Autodesk Inventor part; units mm, degrees
ref_plane "YZ Plane" through (0, 0, 0) normal (1, 0, 0) x (0, 1, 0)
ref_plane "XZ Plane" through (0, 0, 0) normal (0, 1, 0) x (-1, 0, 0)
ref_plane "XY Plane" through (0, 0, 0) normal (0, 0, 1) x (1, 0, 0)
sketch "Sketch1" plane through (0, 0, 0) normal (0, 0, 1) x (1, 0, 0)
  circle A0 centre (0, 0) radius 15.25
  circle A1 centre (0, 0) radius 17.5
  line L0 (-17.4453, -1.3829) -> (-17.4453, 0)
  line L1 (-17.9063, 7.789) -> (-15.9453, 7.789)
  line L2 (-15.9453, 7.789) -> (-15.9453, -7.211)
  line L3 (-15.9453, -7.211) -> (-17.9063, -7.211)
  line L4 (-17.9063, -7.211) -> (-17.9063, 7.789)
  line L5 (-17.9063, 7.789) -> (-15.9453, 7.789)
  line L6 (-15.9453, 7.789) -> (-15.9453, -7.211)
  line L7 (-15.9453, -7.211) -> (-17.9063, -7.211)
  line L8 (-17.9063, -7.211) -> (-17.9063, 7.789)
  point P0 (-15.9453, 0.289)
  dimension "d0" = 30.5
  dimension "d1" = 35
  dimension "d20" = 1.5
extrude "Extrusion1" add sketch "Sketch1" along normal blind 110 contours A1 L2 | L2 A1
sketch "Sketch4" plane through (0, 0, 110) normal (0, 0, 1) x (1, 0, 0)
  circle A0 centre (0, 0) radius 17.5
  point P0 (17.5, 0)
sketch "Sketch6" plane through (0, 0, 110) normal (0, 0, 1) x (1, 0, 0)
  line L0 (-22.5, 7) -> (-12.5, 7)
  line L1 (-12.5, 7) -> (-12.5, -8)
  line L2 (-12.5, -8) -> (-22.5, -8)
  line L3 (-22.5, -8) -> (-22.5, 7)
  circle A0 centre (0, 0) radius 17.5
  dimension "d21" = 5
  dimension "d24" = 10
extrude "Extrusion4" cut sketch "Sketch6" against normal through all contours L0 A0 L2 L3 | L0 L1 L2 A0 picked at (-14.1637, -0.5178)
ref_plane "Work Plane2" through (17.5, 0, 110) normal (1, 0, 0) x (0, 1, 0)
sketch "Sketch7" plane through (17.5, 0, 110) normal (1, 0, 0) x (0, 1, 0)
  circle A0 centre (0, -10) radius 2
  circle A1 centre (0, -90) radius 2
  line L0 (17.5, 0) -> (-17.5, 0)
  point P0 (0, -110)
  point P1 (-8, 0)
  point P2 (7, 0)
  point P3 (0, 0)
  dimension "d25" = 10
  dimension "d26" = 80
  dimension "d27" = 4
  dimension "d28" = 4
extrude "Extrusion5" cut sketch "Sketch7" against normal blind 10
equation "\"BendRadius\" = Thickness"
equation "\"BendReliefWidth\" = Thickness"
equation "\"BendReliefDepth\" = 0.5 * Thickness"
equation "\"CornerReliefSize\" = 4 * Thickness"
equation "\"MinimumRemnant\" = 2 * Thickness"
equation "\"TransitionRadius\" = BendRadius"
equation "\"JacobiRadiusSize\" = BendRadius"
equation "\"GapSize\" = Thickness"
properties part number "Solenoid Yoke"
Source: CAD feature listing. Evaluate the final solid. Frame: model axes, mm. A direction names the side the tool comes from. Give positions to 0.01 mm unless a question says otherwise; leave off trailing zeros. Order: outer loops, then holes, each group sorted by start corner. A loop starts at its lowest first (then second) coordinate and runs counter-clockwise, first axis right, second up.
(1) Access query for faces 1 (the face through (-15, 7, 56)), 2 (the face through (16, 0, 22)). Directions: +Z, -Z, +X, -X, +Y, -Y. A direction counts if a zero-diameter tool reaches every point of the face in a straight line with its end or side. Return the directions, or none.
(2) Pull-direction query (Y, two-part tool) for faces 3 (the face through (16, 0, 102)), 4 (the face through (17.46, 1.21, 54.23)), 5 (the face through (16, 0, 110)); classes: +Y half, -Y half, draft (parallel to the pull), parting line (faces both ways), or undercut.
(3) Section query A-A (x = 0). Return the cut outline in (y, z), plus the area to 3 significant figures.
(4) Section query C-C (z = 20). Return the cut outline in (x, y).
(5) Material intervals for line 1 along Z through (x, y) = (16, 0); line 2 along Y through (x, z) = (0, 84); line 3 along Y through (x, z) = (5, 47.5), sorted ascending.
(6) Contact query for flat-ended pins moving along their axis: P1, Ø1.5, axis at y = -3, z = 42, coming from the -X side; P2, Ø1.5, axis at x = -1, z = 24.5, coming from the +Y side; P3, Ø1.3, axis at x = -14.5, z = 73.5, coming from the +Y side; P4, Ø3, axis at y = 0, z = 20, coming from the +X side. Output: stop coordinate, or through.
(7) Section query D-D (z = 44.5). Return the cut outline in (x, y).
(8) Section query B-B (y = 0). Return the cut outline in (x, z), plus the area to 4 significant figures.
Outcome:
1. face 1: +Z, -Z, -X
1. face 2: +X, -X
2. face 3: undercut
2. face 4: parting line
2. face 5: draft
3. outline: (-17.5, 0) - (-15.25, 0) - (-15.25, 110) - (-17.5, 110) - close; (15.25, 0) - (17.5, 0) - (17.5, 110) - (15.25, 110) - close
3. area: 495 mm2
4. outline: (-16.04, 7) - (-13.55, 7) arc R15.25 cw to (15.12, 2) - (17.39, 2) arc R17.5 ccw to start; (-15.56, -8) arc R17.5 ccw to (17.39, -2) - (15.12, -2) arc R15.25 cw to (-12.98, -8) - close
5. line 1: z = 0 to 18, 22 to 98, 102 to 110
5. line 2: y = -17.5 to -15.25, 15.25 to 17.5
5. line 3: y = -16.77 to -14.41, 14.41 to 16.77
6. P1: stops at x = 14.78
6. P2: stops at y = 17.5
6. P3: stops at y = 10.7
6. P4: passes through
7. outline: (-16.04, 7) - (-13.55, 7) arc R15.25 cw (long way) to (-12.98, -8) - (-15.56, -8) arc R17.5 ccw (long way) to start
8. outline: (15.25, 0) - (17.5, 0) - (17.5, 18) - (15.25, 18) - close; (15.25, 22) - (17.5, 22) - (17.5, 98) - (15.25, 98) - close; (15.25, 102) - (17.5, 102) - (17.5, 110) - (15.25, 110) - close
8. area: 229.5 mm2
